Geometry: final body of the model. Coordinates: model frame, mm. Face numbers are marked on the shaded views. Give positions to 0.01 mm unless a question says otherwise; leave off trailing zeros. Loops run counter-clockwise (first coordinate to the right, second up) from the corner with the lowest first, then second, coordinate; pieces in that order, holes last. Notation, with made-up numbers: (-4.75, 81) -> (39.25, 81) arc R10 ccw to (39.25, 86) -> close; hole circle Ø7 at (29.5, 70). An arc over 180 degrees is marked (long way). One line per item, written item: value. Start each with the question number.
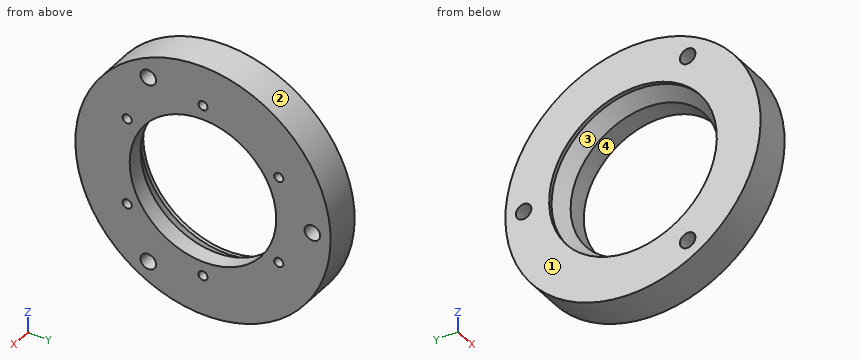
from build123d import *

# Parameters (mm, degrees)
F2_R            = 4.25
F3_DEPTH        = 20.001
F3_COPIES_COUNT = 3
F5_DEPTH        = 15
F5_COPIES_COUNT = 6


# Not quite as in the source:
# - a fillet or chamfer that OpenCascade refuses, or shapes differently, is made with other operations: its cross-section is extruded or revolved along the edge and cut away or added
# - a pattern or mirror of a feature is missing from the dataset's text; its kind, count and spacing are read off the source's solid


with BuildPart() as f1:
    # F0 (on Front) → F1 (revolve)
    with BuildSketch(Plane.XZ):
        Polygon((-10, 40.8116262015), (0, 40.2), (0, 70), (-20, 70), (-20, 46), (-18, 46), align=None)
    revolve(axis=Axis((12.3917190358, 0, 0), (1, 0, 0)))

    # F2 (on face) → F3 (cut, through all)
    with BuildSketch(Plane(origin=(-20, 0, 0), x_dir=(0, -1, 0), z_dir=(-1, 0, 0))):
        with Locations((-60, 0)):
            Circle(F2_R)
    f3 = extrude(amount=-F3_DEPTH, mode=Mode.SUBTRACT)

    # F3_copies: F3 ×3 about axis
    f3_copies_axis = Axis((0, 0, 0), (1, 0, 0))
    for i in range(1, F3_COPIES_COUNT):
        add(f3.rotate(f3_copies_axis, i * 360 / F3_COPIES_COUNT), mode=Mode.SUBTRACT)

    # F4 (on face) → F5 (cut)
    with BuildSketch(Plane.YZ):
        with BuildLine():
            ThreePointArc((-39.0692193817, 24), (-43.9840339474, 24.6470476128), (-39.4041558722, 22.75))
            ThreePointArc((-39.4041558722, 22.75), (-39.1544048159, 23.3529523872), (-39.0692193817, 24))
        make_face()
    f5 = extrude(amount=-F5_DEPTH, mode=Mode.SUBTRACT)

    # F5_copies: F5 ×6 about axis
    f5_copies_axis = Axis((0, 0, 0), (1, 0, 0))
    for i in range(1, F5_COPIES_COUNT):
        add(f5.rotate(f5_copies_axis, i * 360 / F5_COPIES_COUNT), mode=Mode.SUBTRACT)

    # F6: chamfer of 2.5 x 1.5021515476 on 6 edges, made by hand

    # F6_s1 → F6_t2 (revolve)
    with BuildSketch(Plane(origin=(0, 0, 0), x_dir=(1, 0, 0), z_dir=(0, -0.5, -0.8660254038))):
        Polygon((-13.4978484524, 45.5), (-15, 48), (-15, 45.5), align=None)
    revolve(axis=Axis((-15, -41.5692193817, 24), (1, 0, 0)))

    # F6_s3 → F6_t4 (revolve)
    with BuildSketch(Plane(origin=(0, 0, 0), x_dir=(1, 0, 0), z_dir=(0, -0.5, 0.8660254038))):
        Polygon((-13.4978484524, 45.5), (-15, 48), (-15, 45.5), align=None)
    revolve(axis=Axis((-15, 41.5692193817, 24), (1, 0, 0)))

    # F6_s5 → F6_t6 (revolve)
    with BuildSketch(Plane(origin=(0, 0, 0), x_dir=(1, 0, 0), z_dir=(0, 0.5, 0.8660254038))):
        Polygon((-13.4978484524, 45.5), (-15, 48), (-15, 45.5), align=None)
    revolve(axis=Axis((-15, 41.5692193817, -24), (1, 0, 0)))

    # F6_s7 → F6_t8 (revolve)
    with BuildSketch(Plane.XZ):
        Polygon((-13.4978484524, 45.5), (-15, 48), (-15, 45.5), align=None)
    revolve(axis=Axis((-15, 0, 48), (1, 0, 0)))

    # F6_s9 → F6_t10 (revolve)
    with BuildSketch(Plane.XZ):
        Polygon((-13.4978484524, -45.5), (-15, -48), (-15, -45.5), align=None)
    revolve(axis=Axis((-15, 0, -48), (1, 0, 0)))

    # F6_s11 → F6_t12 (revolve)
    with BuildSketch(Plane(origin=(0, 0, 0), x_dir=(1, 0, 0), z_dir=(0, 0.5, -0.8660254038))):
        Polygon((-13.4978484524, 45.5), (-15, 48), (-15, 45.5), align=None)
    revolve(axis=Axis((-15, -41.5692193817, -24), (1, 0, 0)))


solid = f1.part
Item 1: Section A-A, the plane z = 0. Output: boundary loops of the cut face in (x, y), then the cut area to 3 significant figures.
Item 2: Section B-B, the plane x = -4.75. State how many separate pieces and enclosed holes the cut face has, then the cut area to 3 significant figures.
Item 3: Mould query, pull axis Z, two halves, no side actions, for the marked faces 1, 2, 3 and 4. Classes: pulls with the +Z half, pulls with the -Z half, needs draft (parallel to the pull), parting line crosses it, or undercut.
Item 4: Section C-C, the plane y = 60. Output: boundary loops of the cut face in (x, z), then the cut area to 3 significant figures.
Item 5: Pin query (flat end, axial travel): pin 1 (3 mm diameter, centred on y = -41.57, z = 24, fed in from +X); pin 2 (1 mm diameter, centred on x = -17, z = -18, fed in from +Y); pin 3 (13.5 mm diameter, centred on y = -30, z = -51.96, fed in from -X); pin 4 (1 mm diameter, centred on x = -7, z = 41.5, fed in from -Y). Return the tip coordinate at first contact, or that it passes through.
Item 6: Ray query, line 1 along Z through (x, y) = (-9.75, 0); line 2 along Z through (x, y) = (-19.55, 0); line 3 along Y through (x, z) = (-2.75, 24). Return the intervals inside material, ascending. Write a range as [from, to].
Item 7: Section D-D, the plane z = 59.5. Output: boundary loops of the cut face in (x, y).
Geometry check:
1. outline: (-20, -70) -> (0, -70) -> (0, -40.2) -> (-10, -40.81) -> (-18, -46) -> (-20, -46) -> close; (-20, 46) -> (-18, 46) -> (-10, 40.81) -> (0, 40.2) -> (0, 55.75) -> (-20, 55.75) -> close; (-20, 64.25) -> (0, 64.25) -> (0, 70) -> (-20, 70) -> close
1. area: 941 mm2
2. separate pieces: 1
2. enclosed holes: 10
2. area: 9,960 mm2
3. face 1: needs draft
3. face 2: parting line crosses it
3. face 3: undercut
3. face 4: undercut
4. outline: (-20, -36.06) -> (0, -36.06) -> (0, -4.25) -> (-20, -4.25) -> close; (-20, 4.25) -> (0, 4.25) -> (0, 36.06) -> (-20, 36.06) -> close
4. area: 1,270 mm2
5. pin 1: stops at x = -14.1
5. pin 2: stops at y = 67.78
5. pin 3: stops at x = -20
5. pin 4: stops at y = -56.74
6. line 1: z = [-70, -50.5], [-45.5, -40.8], [40.8, 45.5], [50.5, 70]
6. line 2: z = [-70, -46], [46, 70]
6. line 3: y = [-65.76, -44.07], [-39.07, -32.46], [32.46, 39.07], [44.07, 65.76]
7. outline: (-20, -36.87) -> (0, -36.87) -> (0, 36.87) -> (-20, 36.87) -> close
